Autodesk Inventor part; units mm, degrees
ref_plane "YZ Plane" through (0, 0, 0) normal (1, 0, 0) x (0, 1, 0)
ref_plane "XZ Plane" through (0, 0, 0) normal (0, 1, 0) x (-1, 0, 0)
ref_plane "XY Plane" through (0, 0, 0) normal (0, 0, 1) x (1, 0, 0)
sketch "Sketch1" plane through (0, 0, 0) normal (0, 1, 0) x (-1, 0, 0)
  line L0 (0, 0) -> (-11.1125, 9.525)
  line L1 (-11.1125, 9.525) -> (-23.8125, 9.525)
  line L2 (-23.8125, 9.525) -> (-23.8125, 0)
  line L3 (-23.8125, 0) -> (0, 0)
  dimension "plungerWidth" = 9.525
  dimension "plungerLength" = 12.7
  dimension "latchLength" = 11.1125
extrude "Extrusion1" add sketch "Sketch1" against normal blind 12.7
sketch "Sketch2" plane through (23.8125, 0, 9.525) normal (1, 0, 0) x (0, 0, -1)
  circle A0 centre (4.7625, -6.35) radius 1.27
  line L0 (0, 0) -> (9.525, 0)
  line L1 (0, 0) -> (0, -12.7)
  dimension "screwDiameter" = 2.54
  dimension "d8" = 6.35
  dimension "d9" = 4.7625
extrude "Extrusion2" cut sketch "Sketch2" against normal blind 12.7
equation "\"d8\" = 0.5 * plungerHeight"
equation "\"d9\" = 0.5 * plungerWidth"
equation "\"screwDepth\" = plungerLength"
equation "\"plungerTolerance\" = 1.5875"
properties part number "BatteryLatch-Latch"
Geometry check sheet. Reference: the model listing, model coordinates, mm. A direction names the side the tool comes from. Give positions to 0.01 mm unless a question says otherwise; leave off trailing zeros. Loops run counter-clockwise (first coordinate to the right, second up) from the corner with the lowest first, then second, coordinate; pieces in that order, holes last. Notation, with made-up numbers: (27, 3) -> (52, 3) arc R25 ccw to (52, 34) -> close; hole circle Ø8 at (31, -12.75). An arc over 180 degrees is marked (long way). Answer in a Markdown table with one row per item. Add a question column.
1) Draft check along Z on faces 1 (the face through (5.478, -6.261, 4.696)), 2 (the face through (17.55, -5.97, 3.55)), 3 (the face through (12, -6, 0)). Enter one of: pulls with the +Z half, pulls with the -Z half, needs draft (parallel to the pull), parting line crosses it, or undercut.
2) Set-up check for faces 4 (the face through (23.812, -8, 5)), 5 (the face through (11.112, -6, 5)): record each of +Z, -Z, +X, -X, +Y, -Y from which the full face is reachable in a straight line by a thin tool's end or side.
3) Material ranges on probe 1 along Y at (x, z) = (22.25, 3.75); probe 2 along Y at (x, z) = (18, 4.25); probe 3 along Z at (x, y) = (22.25, -7) (3 decimals), recorded low to high. Write a range as from..to.
4) Cross-section at B-B on y = -6.35. Record the boundary of the cut face in (x, z) (1 decimal).
5) Cross-section at C-C on z = 7.5. Record the boundary of the cut face in (x, y), and give its area (3 significant figures).
6) Cross-section at D-D on x = 1.75. Record the boundary of the cut face in (y, z).
7) Gauge pin test, flat ends, axial feed: P1, Ø3, axis at y = -9, z = 2, coming from the -X side; P2, Ø6, axis at x = 5.5, y = -5, coming from the +Z side; P3, Ø0.8, axis at y = -6, z = 5, coming from the +X side. Record the tip position at first contact, or that the pin passes through.
Outcome:
| question | item | result |
|---|---|---|
| 1 | face 1 | pulls with the +Z half |
| 1 | face 2 | undercut |
| 1 | face 3 | pulls with the -Z half |
| 2 | face 4 | +Z, -Z, +X, +Y, -Y |
| 2 | face 5 | +X |
| 3 | probe 1 | y = -12.7..-7.12, -5.58..0 |
| 3 | probe 2 | y = -12.7..-7.51, -5.19..0 |
| 3 | probe 3 | z = 0..3.671, 5.854..9.525 |
| 4 | outline | (0, 0) -> (23.8, 0) -> (23.8, 3.5) -> (11.1, 3.5) -> (11.1, 6) -> (23.8, 6) -> (23.8, 9.5) -> (11.1, 9.5) -> close |
| 5 | outline | (8.75, -12.7) -> (23.81, -12.7) -> (23.81, 0) -> (8.75, 0) -> close |
| 5 | area | 191 mm^2 |
| 6 | outline | (-12.7, 0) -> (0, 0) -> (0, 1.5) -> (-12.7, 1.5) -> close |
| 7 | P1 | stops at x = 0.58 |
| 7 | P2 | stops at z = 7.29 |
| 7 | P3 | stops at x = 11.11 |
